Check sheet for the modelled part. Datum: model origin and axes. Units: mm. Face numbers are marked on the shaded views. A direction names the side the tool comes from. Coordinates: 2 decimals unless noted, no trailing zeros. Write each loop counter-clockwise with the first axis right and the second up, starting at its lowest first coordinate (ties: lowest second). Pieces come first, ordered by that corner, then holes. Notation, with made-up numbers: (36.5, -32.75) -> (70.5, -32.75) arc R32 cw to (70.5, 0.25) -> close; hole circle Ø5 at (15.25, 23). An arc over 180 degrees is marked (long way). Put each result on its own line as item: value.
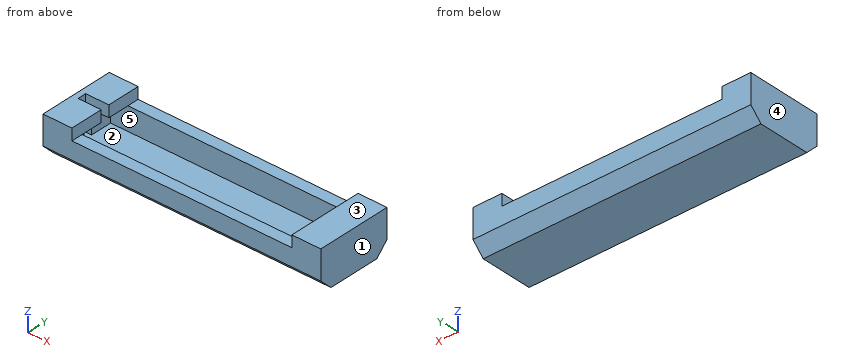
```python
from build123d import *

# Parameters (mm, degrees)
F0_W     = 48
F0_H     = 13
F0_W_2   = 44
F0_H_2   = 9
F1_DEPTH = 4
F2_DEPTH = 1
F3_W     = 3
F3_H     = 9
F4_DEPTH = 2
F5_SIZE  = 2
F6_W     = 1.5
F6_H     = 6
F7_DEPTH = 4


with BuildPart() as f1:
    # F0 (on Top) → F1 (new body)
    with BuildSketch(Plane.XY):
        Rectangle(F0_W, F0_H)
        Rectangle(F0_W_2, F0_H_2, mode=Mode.SUBTRACT)
    extrude(amount=F1_DEPTH)

    # F0 (on Top) → F2 (join)
    with BuildSketch(Plane.XY):
        Rectangle(F0_W, F0_H)
        Rectangle(F0_W_2, F0_H_2, mode=Mode.SUBTRACT)
        Rectangle(F0_W_2, F0_H_2)
    extrude(amount=-F2_DEPTH)

    # F3 (on face) → F4 (join)
    with BuildSketch(Plane.XY.offset(4)):
        Polygon((-19, 4.5), (-19, 6.5), (-24, 6.5), (-24, -6.5), (-19, -6.5), (-19, -4.5), (-22, -4.5), (-22, 4.5), align=None)
        with Locations((-20.5, 0)):
            Rectangle(F3_W, F3_H)
        Polygon((24, 6.5), (19, 6.5), (19, 4.5), (22, 4.5), (22, -4.5), (19, -4.5), (19, -6.5), (24, -6.5), align=None)
        with Locations((20.5, 0)):
            Rectangle(F3_W, F3_H)
    extrude(amount=F4_DEPTH)

    # F5
    f5_edges = [f1.edges().sort_by_distance(p)[0] for p in [
        (0, -6.5, -1),
        (0, 6.5, -1),
    ]]
    chamfer(f5_edges, length=F5_SIZE)

    # F6 (on face) → F7 (cut)
    with BuildSketch(Plane.YZ.offset(-19)):
        with Locations((0, 3)):
            Rectangle(F6_W, F6_H)
    extrude(amount=-F7_DEPTH, mode=Mode.SUBTRACT)


solid = f1.part
```
Q1. Cross-section at A-A (z = 5). Record the cut outline in (x, y), plus the area to 3 significant figures.
Recorded:
outline: (-24, -6.5) -> (-19, -6.5) -> (-19, -0.75) -> (-23, -0.75) -> (-23, 0.75) -> (-19, 0.75) -> (-19, 6.5) -> (-24, 6.5) -> close; (19, -6.5) -> (24, -6.5) -> (24, 6.5) -> (19, 6.5) -> close
area: 124 mm2
Q2. Depth check by flat-ended pin: P1, Ø2, axis at x = 4.5, y = -5.5, coming from the +Z side; P2, Ø2.5, axis at x = 0.5, y = 2, coming from the +Z side. Enter the tip coordinate at first touch or a pass-through.
Recorded:
P1: stops at z = 4
P2: stops at z = 0
Q3. Cross-section at C-C (z = 2.25). Record the cut outline in (x, y), plus the area to 4 significant figures.
Recorded:
outline: (-24, -6.5) -> (24, -6.5) -> (24, 6.5) -> (-24, 6.5) -> close; hole (-23, -0.75) -> (-22, -0.75) -> (-22, -4.5) -> (22, -4.5) -> (22, 4.5) -> (-22, 4.5) -> (-22, 0.75) -> (-23, 0.75) -> close
area: 226.5 mm2
Q4. Cross-section at D-D (x = -9). Record the cut outline in (y, z).
Recorded:
outline: (-6.5, 1) -> (-4.5, -1) -> (4.5, -1) -> (6.5, 1) -> (6.5, 4) -> (4.5, 4) -> (4.5, 0) -> (-4.5, 0) -> (-4.5, 4) -> (-6.5, 4) -> close
Q5. Material ranges on line 1 along Y through (x, z) = (2, 1.5); line 2 along X through (y, z) = (-1.5, 1.75); line 3 along X through (y, z) = (-5.25, 4.5), recorded low to high.
Recorded:
line 1: y = -6.5 to -4.5, 4.5 to 6.5
line 2: x = -24 to -22, 22 to 24
line 3: x = -24 to -19, 19 to 24
Q6. Mould release check, pull along X, two halves, no side actions. Record for the marked faces 1, 2 and 3: released by +X, released by -X, zero draft, split by the parting line, or undercut.
Recorded:
face 1: released by +X
face 2: undercut
face 3: zero draft
Q7. Cross-section at B-B (y = 1.5). Record the cut outline in (x, z).
Recorded:
outline: (-24, -1) -> (24, -1) -> (24, 6) -> (19, 6) -> (19, 4) -> (22, 4) -> (22, 0) -> (-22, 0) -> (-22, 4) -> (-19, 4) -> (-19, 6) -> (-24, 6) -> close
Q8. Tool access check on the marked faces 4 and 5. Record the directions out of +Z, -Z, +X, -X, +Y, -Y that give a thin tool (end or side, any length) a straight path to the whole face; none if there is none.
Recorded:
face 4: +Z, -Z, -X, +Y, -Y
face 5: none
